Work out the finished part from the listing and answer in its coordinate system (mm). A direction names the side the tool comes from. Give positions to 0.01 mm unless a question says otherwise; leave off trailing zeros. Write each loop counter-clockwise with the first axis right and the second up, starting at its lowest first coordinate (ties: lowest second). Pieces come first, ordered by that corner, then holes.
1) Find section C-C (x = -22.5). Determine the outline of the cut face in (y, z), plus the area to 3 significant figures.
2) Find section A-A (y = 27.5). Determine the outline of the cut face in (x, z) (3 decimals), plus the area to 3 significant figures.
3) Straight lines are drawn through the part: probe 1 along Z at (x, y) = (-11.75, 22); probe 2 along Y at (x, z) = (-4.75, -11); probe 3 along X at (y, z) = (5.25, 0) (3 decimals). For each, find the intervals that lie inside material, in ascending order.
4) Find section D-D (x = -19). Determine the outline of the cut face in (y, z), plus the area to 3 significant figures.
5) Find section B-B (z = 0). Determine the outline of the cut face in (x, y) (3 decimals), plus the area to 3 significant figures.
6) Determine the mould class of faces 1 (the face through (-16, 25, -12.7)), 2 (the face through (-16.154, 44.447, 15.919)), 3 (the face through (-16, 22, 19.05)) for opening direction Z: pulls with the +Z half, pulls with the -Z half, needs draft (parallel to the pull), parting line crosses it, or undercut.
7) A tool of negligible diameter and unlimited length cuts with its end or side. For faces 4 (the face through (-16, 22, -19.05)), 5 (the face through (-19, 6.35, -3)), from which of +Z, -Z, +X, -X, +Y, -Y can it reach the whole face along a straight path? Write none if from no direction.
8) Given pin 1 Ø6 at (x, z) = (-21, 11) entering from +Y; pin 2 Ø6 at (x, z) = (-23.5, -3) entering from +Y; pin 3 Ø6 at (y, z) = (32, -8.5) entering from -X, each flat-ended and moving along its own axis, determine where each tip first touches the part or whether it passes through.
```python
from build123d import *

# Parameters (mm, degrees)
SKETCH1_W           = 57.15
SKETCH1_H           = 38.1
BOSS_EXTRUDE1_DEPTH = 50.8
SKETCH4_W           = 25.4
SKETCH4_H           = 44.45
CUT_EXTRUDE2_DEPTH  = 79.801427652
SKETCH2_R           = 3.175
CUT_EXTRUDE1_DEPTH  = 70.633186233
SKETCH5_R           = 3.96875
CUT_EXTRUDE3_DEPTH  = 57.171484091


with BuildPart() as part:
    # Sketch1 → Boss-Extrude1 (new body)
    with BuildSketch(Plane(origin=(0, 0, 0), x_dir=(1, 0, 0), z_dir=(0, 1, 0))):
        Rectangle(SKETCH1_W, SKETCH1_H)
    extrude(amount=BOSS_EXTRUDE1_DEPTH)

    # Sketch4 → Cut-Extrude2 (cut, through all)
    with BuildSketch(Plane.ZY.offset(28.575)):
        with Locations((0, 28.575)):
            Rectangle(SKETCH4_W, SKETCH4_H)
    extrude(amount=-CUT_EXTRUDE2_DEPTH, mode=Mode.SUBTRACT)

    # Sketch2 → Cut-Extrude1 (cut, through all)
    with BuildSketch(Plane.XY.offset(19.05)):
        with BuildLine():
            Line((-3.175, 0), (28.575, 0))
            Line((28.575, 0), (28.575, 50.8))
            Line((28.575, 50.8), (-28.575, 50.8))
            Line((-28.575, 50.8), (-28.575, 31.75))
            ThreePointArc((-28.575, 31.75), (-15.875, 44.45), (-3.175, 31.75))
            Line((-3.175, 31.75), (-3.175, 0))
        make_face()
        with Locations((-19.84375, 36.5125)):
            Circle(SKETCH2_R)
    extrude(amount=-CUT_EXTRUDE1_DEPTH, mode=Mode.SUBTRACT)

    # Sketch5 → Cut-Extrude3 (cut, through all)
    with BuildSketch(Plane.XZ):
        with Locations(Location((-15.875, 0, 0), (0, 0, 270))):
            Circle(SKETCH5_R)
    extrude(amount=-CUT_EXTRUDE3_DEPTH, mode=Mode.SUBTRACT)


solid = part.part
```
Results:
1. outline: (0, -19.05) - (34.77, -19.05) - (34.77, -12.7) - (6.35, -12.7) - (6.35, 12.7) - (34.77, 12.7) - (34.77, 19.05) - (0, 19.05) - close; (38.25, -19.05) - (42.59, -19.05) - (42.59, -12.7) - (38.25, -12.7) - close; (38.25, 12.7) - (42.59, 12.7) - (42.59, 19.05) - (38.25, 19.05) - close
1. area: 658 mm2
2. outline: (-28.575, -19.05) - (-3.175, -19.05) - (-3.175, -12.7) - (-28.575, -12.7) - close; (-28.575, 12.7) - (-3.175, 12.7) - (-3.175, 19.05) - (-28.575, 19.05) - close
2. area: 323 mm2
3. probe 1: z = -19.05 to -12.7, 12.7 to 19.05
3. probe 2: y = 0 to 6.35
3. probe 3: x = -28.575 to -19.844, -11.906 to -3.175
4. outline: (0, -19.05) - (33.45, -19.05) - (33.45, -12.7) - (6.35, -12.7) - (6.35, -2.45) - (0, -2.45) - close; (0, 2.45) - (6.35, 2.45) - (6.35, 12.7) - (33.45, 12.7) - (33.45, 19.05) - (0, 19.05) - close; (39.57, -19.05) - (44.06, -19.05) - (44.06, -12.7) - (39.57, -12.7) - close; (39.57, 12.7) - (44.06, 12.7) - (44.06, 19.05) - (39.57, 19.05) - close
4. area: 612 mm2
5. outline: (-28.575, 0) - (-19.844, 0) - (-19.844, 6.35) - (-28.575, 6.35) - close; (-11.906, 0) - (-3.175, 0) - (-3.175, 6.35) - (-11.906, 6.35) - close
5. area: 111 mm2
6. face 1: undercut
6. face 2: needs draft
6. face 3: pulls with the +Z half
7. face 4: -Z, +X, -X, +Y, -Y
7. face 5: +X, -X, +Y
8. pin 1: stops at y = 44.17
8. pin 2: stops at y = 6.35
8. pin 3: passes through
